Check sheet for the modelled part. Datum: model origin and axes. Units: mm. Face numbers are marked on the shaded views. A direction names the side the tool comes from. Round coordinates to 2 decimals unless told otherwise and drop trailing zeros. Loops run counter-clockwise (first coordinate to the right, second up) from the corner with the lowest first, then second, coordinate; pieces in that order, holes last. Notation, with made-up numbers: (42.25, 5) - (60.25, 5) arc R24 cw to (60.25, 24) - close; hole circle Ø3 at (34.5, 53.5). An arc over 180 degrees is marked (long way). Answer in a Markdown table with one row per item. Add a question column.
(1) Thickness scan on line 1 along X through (y, z) = (3.85, -18); line 2 along X through (y, z) = (5.65, 6.5). Record the ranges inside material, lowest first.
(2) Cross-section at C-C on y = 0.8. Enter the section's corners in (x, z).
(3) Cross-section at A-A on z = 18. Enter the section's corners in (x, y), then the cut area to 3 significant figures.
(4) Gauge pin test, flat end, axial feed: pin 1 (6 mm diameter, centred on x = -4, z = -6.5, fed in from +Y). Record the tip position at first contact, or that the pin passes through.
(5) Cross-section at B-B on x = 0. Enter the section's corners in (y, z), then the cut area to 3 significant figures.
(6) Mould release check, pull along X, two halves, no side actions. Record for the marked faces 1, 2, 3 and 4: +X half, -X half, draft (parallel to the pull), parting line (faces both ways), or undercut.
(7) Cross-section at D-D on z = 0. Enter the section's corners in (x, y), then the cut area to 3 significant figures.
(8) Access from +Z, -Z, +X, -X, +Y, -Y to the whole of each face (thin tool, end or side, straight path). Record for the marked faces 5 and 6.
from build123d import *

# Parameters (mm, degrees)
IZIM1_R                     = 7.1
IZIM1_R_2                   = 2
Y_KSEKLIK_EKSTR_ZYON1_DEPTH = 5.8
KES_EKSTR_ZYON1_DEPTH       = 1


with BuildPart() as part:
    # Çizim1 → Yükseklik-Ekstrüzyon1 (new body)
    with BuildSketch(Plane(origin=(0, 0, 0), x_dir=(1, 0, 0), z_dir=(0, 1, 0))):
        with BuildLine():
            Line((-20.15, -24.15), (20.15, -24.15))
            ThreePointArc((20.15, -24.15), (22.978427125, -22.978427125), (24.15, -20.15))
            Line((24.15, -20.15), (24.15, 20.15))
            ThreePointArc((24.15, 20.15), (22.978427125, 22.978427125), (20.15, 24.15))
            Line((20.15, 24.15), (-20.15, 24.15))
            ThreePointArc((-20.15, 24.15), (-22.978427125, 22.978427125), (-24.15, 20.15))
            Line((-24.15, 20.15), (-24.15, -20.15))
            ThreePointArc((-24.15, -20.15), (-22.978427125, -22.978427125), (-20.15, -24.15))
        make_face()
        Circle(IZIM1_R, mode=Mode.SUBTRACT)
        with Locations((-18, 18)):
            Circle(IZIM1_R_2, mode=Mode.SUBTRACT)
        with Locations((-18, -18)):
            Circle(IZIM1_R_2, mode=Mode.SUBTRACT)
        with Locations((18, -18)):
            Circle(IZIM1_R_2, mode=Mode.SUBTRACT)
        with Locations((18, 18)):
            Circle(IZIM1_R_2, mode=Mode.SUBTRACT)
    extrude(amount=Y_KSEKLIK_EKSTR_ZYON1_DEPTH)

    # Çizim2 → Kes-Ekstrüzyon1 (cut)
    with BuildSketch(Plane(origin=(0, 5.8, 0), x_dir=(1, 0, 0), z_dir=(0, 1, 0))):
        with BuildLine():
            Line((-20.9, -22.9), (20.9, -22.9))
            ThreePointArc((20.9, -22.9), (22.314213562, -22.314213562), (22.9, -20.9))
            Line((22.9, -20.9), (22.9, 20.9))
            ThreePointArc((22.9, 20.9), (22.314213562, 22.314213562), (20.9, 22.9))
            Line((20.9, 22.9), (-20.9, 22.9))
            ThreePointArc((-20.9, 22.9), (-22.314213562, 22.314213562), (-22.9, 20.9))
            Line((-22.9, 20.9), (-22.9, -20.9))
            ThreePointArc((-22.9, -20.9), (-22.314213562, -22.314213562), (-20.9, -22.9))
        make_face()
    extrude(amount=-KES_EKSTR_ZYON1_DEPTH, mode=Mode.SUBTRACT)


solid = part.part
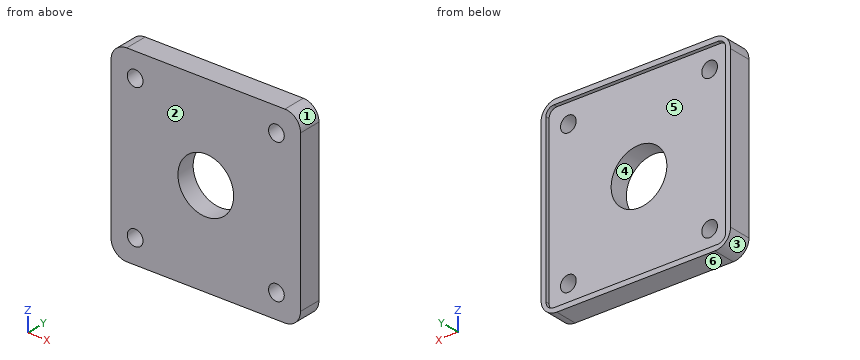
Answers:
| question | item | result |
|---|---|---|
| 1 | line 1 | x = -24.15 to -20, -16 to 16, 20 to 24.15 |
| 1 | line 2 | x = -24.15 to -22.9, 22.9 to 24.15 |
| 2 | outline | (-24.15, -20.15) arc R4 ccw to (-20.15, -24.15) - (20.15, -24.15) arc R4 ccw to (24.15, -20.15) - (24.15, 20.15) arc R4 ccw to (20.15, 24.15) - (-20.15, 24.15) arc R4 ccw to (-24.15, 20.15) - close; hole circle Ø4 at (-18, -18); hole circle Ø4 at (-18, 18); hole circle Ø14.2 at (0, 0); hole circle Ø4 at (18, -18); hole circle Ø4 at (18, 18) |
| 3 | outline | (-24.15, 0) - (-20, 0) - (-20, 4.8) - (-22.9, 4.8) - (-22.9, 5.8) - (-24.15, 5.8) - close; (-16, 0) - (16, 0) - (16, 4.8) - (-16, 4.8) - close; (20, 0) - (24.15, 0) - (24.15, 5.8) - (22.9, 5.8) - (22.9, 4.8) - (20, 4.8) - close |
| 3 | area | 196 mm^2 |
| 4 | pin 1 | stops at y = 4.8 |
| 5 | outline | (0, -24.15) - (5.8, -24.15) - (5.8, -22.9) - (4.8, -22.9) - (4.8, -7.1) - (0, -7.1) - close; (0, 7.1) - (4.8, 7.1) - (4.8, 22.9) - (5.8, 22.9) - (5.8, 24.15) - (0, 24.15) - close |
| 5 | area | 166 mm^2 |
| 6 | face 1 | +X half |
| 6 | face 2 | draft |
| 6 | face 3 | -X half |
| 6 | face 4 | undercut |
| 7 | outline | (-24.15, 0) - (-7.1, 0) - (-7.1, 4.8) - (-22.9, 4.8) - (-22.9, 5.8) - (-24.15, 5.8) - close; (7.1, 0) - (24.15, 0) - (24.15, 5.8) - (22.9, 5.8) - (22.9, 4.8) - (7.1, 4.8) - close |
| 7 | area | 166 mm^2 |
| 8 | face 5 | +Y |
| 8 | face 6 | -Z, +X, -X, +Y, -Y |
